Verification items for the finished model (mm, model axes). A direction names the side the tool comes from. Round coordinates to 2 decimals unless told otherwise and drop trailing zeros. Order: outer loops, then holes, each group sorted by start corner. A loop starts at its lowest first (then second) coordinate and runs counter-clockwise, first axis right, second up. Notation, with made-up numbers: (75, 64) -> (107, 64) arc R22 cw to (107, 70) -> close; hole circle Ø3 at (-28.5, 42.25). An arc over 180 degrees is marked (long way). Put each result on its own line as item: value.
```python
from build123d import *

# Parameters (mm, degrees)
SKETCH1_R                       = 4.05
BOSS_EXTRUDE1_DEPTH             = 8
SKETCH2_W                       = 18.1
SKETCH2_H                       = 4
BOSS_EXTRUDE2_DEPTH             = 33.85
CHAMFER1_SIZE                   = 2.5
CHAMFER1_SIZE_2                 = 9.330127019
CHAMFER2_SIZE                   = 9.330127019
CHAMFER2_SIZE_2                 = 2.5
FILLET1_R                       = 2
SKETCH3_W                       = 18.1
SKETCH3_H                       = 4
BOSS_EXTRUDE3_DEPTH             = 35
CHAMFER3_SIZE                   = 4
F_4_0MM_DOWEL_HOLE1_D           = 4
F_4_0MM_DOWEL_HOLE1_CSINK_D     = 4.05
F_4_0MM_DOWEL_HOLE1_CSINK_ANGLE = 90
FILLET2_R                       = 2
CUT_EXTRUDE1_DEPTH              = 54.698463665
CUT_EXTRUDE1_DEPTH_BACK         = 54.698463665
CUT_EXTRUDE2_DEPTH              = 54.698463665
CUT_EXTRUDE2_DEPTH_BACK         = 54.698463665


with BuildPart() as part:
    # Sketch1 → Boss-Extrude1 (new body)
    with BuildSketch(Plane.XY):
        Circle(SKETCH1_R)
    extrude(amount=BOSS_EXTRUDE1_DEPTH)

    # Sketch2 → Boss-Extrude2 (add)
    with BuildSketch(Plane.XY.offset(8)):
        Rectangle(SKETCH2_W, SKETCH2_H)
    extrude(amount=BOSS_EXTRUDE2_DEPTH)

    # Chamfer1
    # the kernel refuses this chamfer: 9.330127019, 2.5 mm, written as the material it adds along each edge
    with BuildSketch(Plane(origin=(27.749460413, 2, 8), x_dir=(0, 0.9905000388259542, -0.1375124470212913), z_dir=(-1, 0, 0))) as chamfer1_piece_1_section:
        Polygon((CHAMFER1_SIZE * 0.990500038826, -CHAMFER1_SIZE * 0.137512447021), (-CHAMFER1_SIZE_2 * 0.13751244702, -CHAMFER1_SIZE_2 * 0.990500038818), (0, 0), align=None)
    chamfer1_piece_1 = extrude(amount=55.498920827, mode=Mode.PRIVATE)
    chamfer1_piece_1 = chamfer1_piece_1 & Plane(origin=(0, 0, 11.423628779), x_dir=(1, 0, 0), z_dir=(0, 0, -1)) * Cylinder(4.05, 148, mode=Mode.PRIVATE)
    add(chamfer1_piece_1)

    # Chamfer2
    # the kernel refuses this chamfer: 9.330127019, 2.5 mm, written as the material it adds along each edge
    with BuildSketch(Plane(origin=(-27.749460413, -2, 8), x_dir=(0, 0.009967146577156291, 0.9999503267608394), z_dir=(1, 0, 0))) as chamfer2_piece_1_section:
        Polygon((CHAMFER2_SIZE * 0.999950326753, CHAMFER2_SIZE * 0.00996714657707), (-CHAMFER2_SIZE_2 * 0.00996714657716, CHAMFER2_SIZE_2 * 0.999950326761), (0, 0), align=None)
    chamfer2_piece_1 = extrude(amount=55.498920827, mode=Mode.PRIVATE)
    chamfer2_piece_1 = chamfer2_piece_1 & Plane(origin=(0, 0, 11.423628779), x_dir=(1, 0, 0), z_dir=(0, 0, -1)) * Cylinder(4.05, 149, mode=Mode.PRIVATE)
    add(chamfer2_piece_1)

    # Fillet1
    fillet1_edges = [part.edges().sort_by_distance(p)[0] for p in [
        (9.05, 0, 8),
        (-9.05, 0, 8),
    ]]
    fillet(fillet1_edges, radius=FILLET1_R)

    # Sketch3 → Boss-Extrude3 (add)
    with BuildSketch(Plane(origin=(0, 2, 0), x_dir=(1, 0, 0), z_dir=(0, 1, 0))):
        with Locations((0, -39.85)):
            Rectangle(SKETCH3_W, SKETCH3_H)
    extrude(amount=BOSS_EXTRUDE3_DEPTH)

    # Chamfer3
    chamfer3_edges = [part.edges().sort_by_distance(p)[0] for p in [
        (0, 2, 37.85),
    ]]
    chamfer(chamfer3_edges, length=CHAMFER3_SIZE)

    # Ø4.0mm Dowel Hole1 (through all)
    with Locations(Plane.XY.offset(41.85)):
        with Locations((0, 31), (0, 22), (0, 13)):
            CounterSinkHole(F_4_0MM_DOWEL_HOLE1_D / 2, F_4_0MM_DOWEL_HOLE1_CSINK_D / 2, counter_sink_angle=F_4_0MM_DOWEL_HOLE1_CSINK_ANGLE)

    # Fillet2
    fillet2_edges = [part.edges().sort_by_distance(p)[0] for p in [
        (0, -2, 41.85),
    ]]
    fillet(fillet2_edges, radius=FILLET2_R)

    # Sketch6 → Cut-Extrude1 (cut, two sides: drawn at the far end of the back side and taken through both)
    with BuildSketch(Plane(origin=(0, 0, 37.85), x_dir=(-1, 0, 0), z_dir=(0, 0, -1)).offset(-CUT_EXTRUDE1_DEPTH_BACK)):
        Polygon((-9.05, 6), (-5.5, 7.98), (-5.5, 37), (-9.05, 37), align=None)
    extrude(amount=CUT_EXTRUDE1_DEPTH + CUT_EXTRUDE1_DEPTH_BACK, mode=Mode.SUBTRACT)

    # Sketch7 → Cut-Extrude2 (cut, two sides: drawn at the far end of the back side and taken through both)
    with BuildSketch(Plane(origin=(0, 0, 37.85), x_dir=(-1, 0, 0), z_dir=(0, 0, -1)).offset(-CUT_EXTRUDE2_DEPTH_BACK)):
        Polygon((9.05, 6), (5.5, 7.98), (5.5, 37), (9.05, 37), align=None)
    extrude(amount=CUT_EXTRUDE2_DEPTH + CUT_EXTRUDE2_DEPTH_BACK, mode=Mode.SUBTRACT)


solid = part.part
```
Item 1: Sectioned sample at B-B, the plane x = 0. Give the number of separate pieces and of enclosed holes in the cut face, then the cut area to 3 significant figures.
Geometry check:
separate pieces: 4
enclosed holes: 0
area: 322 mm2
Item 2: Depth check by flat-ended pin: pin 1 Ø5 at (x, y) = (0, 31) entering from -Z; pin 2 Ø1.5 at (x, z) = (-1.5, 27.5) entering from -Y; pin 3 Ø1.2 at (y, z) = (23.5, 39.5) entering from +X; pin 4 Ø10 at (y, z) = (30.5, 30) entering from -X. Enter the tip coordinate at first touch or a pass-through.
Geometry check:
pin 1: z = 37.85
pin 2: y = -2
pin 3: x = 5.5
pin 4: through
Item 3: Material ranges on line 1 along Y through (x, z) = (0, 39.3); line 2 along X through (y, z) = (22, 38); line 3 along Y through (x, z) = (2.25, 38), recorded low to high.
Geometry check:
line 1: -2 to 11, 15 to 20, 24 to 29, 33 to 37
line 2: -5.5 to -2, 2 to 5.5
line 3: -2 to 37
Item 4: Sectioned sample at A-A, the plane y = 22. Record the boundary of the cut face in (x, z) (3 decimals).
Geometry check:
outline: (-5.5, 37.85) -> (-2, 37.85) -> (-2, 41.825) -> (-2.025, 41.85) -> (-5.5, 41.85) -> close; (2, 37.85) -> (5.5, 37.85) -> (5.5, 41.85) -> (2.025, 41.85) -> (2, 41.825) -> close
Item 5: Tool access check on faces 1 (the face through (-5.5, 22, 40)), 2 (the face through (-2, 21, 37.85)), 3 (the face through (-0.13, 4.03, 35.88)), 4 (the face through (-4.046, -0.178, 4.693)), 5 (the face through (0, 2, 21)). Record the directions out of +Z, -Z, +X, -X, +Y, -Y that give a thin tool (end or side, any length) a straight path to the whole face; none if there is none.
Geometry check:
face 1: +Z, -Z, -X, +Y
face 2: -Z, +X, -X, +Y
face 3: +X, -X, +Y
face 4: -Z
face 5: +Y
Item 6: Release check for a two-part mould opening along Z. For faces 6 (the face through (0.05, 2.81, 14.3)), 7 (the face through (-9.05, 1, 26)), 8 (the face through (-2, 14, 41.85)) record: pulls with the +Z half, pulls with the -Z half, needs draft (parallel to the pull), parting line crosses it, or undercut.
Geometry check:
face 6: undercut
face 7: needs draft
face 8: pulls with the +Z half
Item 7: Sectioned sample at C-C, the plane z = 34.5. Record the boundary of the cut face in (x, y).
Geometry check:
outline: (-9.05, -2) -> (9.05, -2) -> (9.05, 2.65) -> (-9.05, 2.65) -> close
